Part model, mm, in its own coordinate system. Face numbers are marked on the shaded views. A direction names the side the tool comes from. Coordinates: 2 decimals unless noted, no trailing zeros. Order: outer loops, then holes, each group sorted by start corner. A loop starts at its lowest first (then second) coordinate and runs counter-clockwise, first axis right, second up.
1) Wall check: L1, parallel to Z at x = 0, y = 6; L2, parallel to X at y = 25.75, z = 0 (3 decimals). Give the ranges that are in metal, low to high.
2) Mould opens along Z. For the marked faces 1, 2 and 3 say: +Z half, -Z half, draft (parallel to the pull), parting line (faces both ways), or undercut.
3) Cut at D-D (y = 21.5). List the corners of the cut face in (x, z).
4) Cut at A-A (z = 0). List the corners of the cut face in (x, y) (3 decimals).
5) Tool access for the marked faces 4 and 5: list every direction of +Z, -Z, +X, -X, +Y, -Y with a clear straight run to the whole face (end or side of a thin tool).
6) Cut at B-B (x = 0). List the corners of the cut face in (y, z) (3 decimals), and give its area (3 significant figures).
7) Pin check, flat tips, straight feed: pin 1 Ø12 at (y, z) = (25.5, -17.5) entering from +X; pin 2 Ø2 at (x, z) = (-6.5, -7.5) entering from +Y; pin 3 Ø2 at (y, z) = (20.5, -1.5) entering from -X. Stop position of each tip, or through.
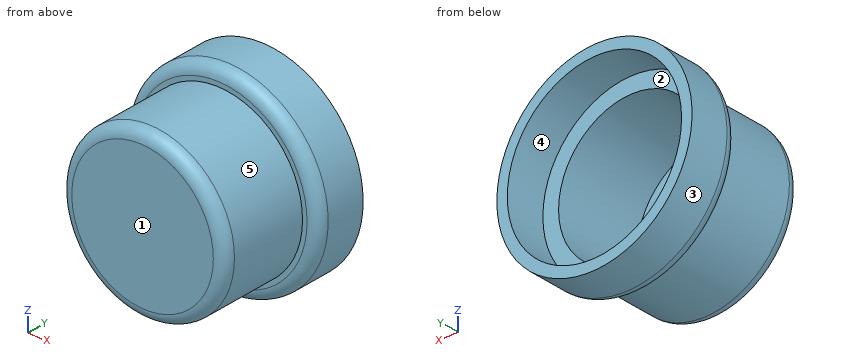
```python
from build123d import *

# Parameters (mm, degrees)
FILLET1_R = 2.54


with BuildPart() as part:
    # Sketch2 → Revolve1 (revolve)
    with BuildSketch(Plane.XY):
        Polygon((0, 0), (18.653125, 0), (18.653125, 19.84375), (22.225, 19.84375), (22.225, 31.27375), (19.84375, 31.27375), (19.84375, 22.225), (16.271875, 22.225), (16.271875, 2.38125), (0, 2.38125), align=None)
    revolve(axis=Axis((0, 0, 0), (0, 1, 0)))

    # Fillet1
    fillet1_edges = [part.edges().sort_by_distance(p)[0] for p in [
        (-18.653125, 0, 0),
        (-22.225, 19.84375, 0),
    ]]
    fillet(fillet1_edges, radius=FILLET1_R)


solid = part.part
```
Geometry check:
1. L1: z = -18.65 to -16.27, 16.27 to 18.65
1. L2: x = -22.225 to -19.844, 19.844 to 22.225
2. face 1: draft
2. face 2: undercut
2. face 3: parting line
3. outline: circle Ø44.13 at (0, 0); hole circle Ø32.54 at (0, 0)
4. outline: (-22.225, 22.384) arc R2.54 ccw to (-19.685, 19.844) - (-18.653, 19.844) - (-18.653, 2.54) arc R2.54 ccw to (-16.113, 0) - (16.113, 0) arc R2.54 ccw to (18.653, 2.54) - (18.653, 19.844) - (19.685, 19.844) arc R2.54 ccw to (22.225, 22.384) - (22.225, 31.274) - (19.844, 31.274) - (19.844, 22.225) - (16.272, 22.225) - (16.272, 2.381) - (-16.272, 2.381) - (-16.272, 22.225) - (-19.844, 22.225) - (-19.844, 31.274) - (-22.225, 31.274) - close
5. face 4: +Y
5. face 5: -Y
6. outline: (0, -16.113) arc R2.54 ccw to (2.54, -18.653) - (19.844, -18.653) - (19.844, -19.685) arc R2.54 ccw to (22.384, -22.225) - (31.274, -22.225) - (31.274, -19.844) - (22.225, -19.844) - (22.225, -16.272) - (2.381, -16.272) - (2.381, 16.272) - (22.225, 16.272) - (22.225, 19.844) - (31.274, 19.844) - (31.274, 22.225) - (22.384, 22.225) arc R2.54 ccw to (19.844, 19.685) - (19.844, 18.653) - (2.54, 18.653) arc R2.54 ccw to (0, 16.113) - close
6. area: 238 mm2
7. pin 1: stops at x = 19.02
7. pin 2: stops at y = 2.38
7. pin 3: stops at x = -22.02
